Geometry check sheet. Reference: the model listing, model coordinates, mm. Round coordinates to 2 decimals unless told otherwise and drop trailing zeros. Order: outer loops, then holes, each group sorted by start corner. A loop starts at its lowest first (then second) coordinate and runs counter-clockwise, first axis right, second up.
```python
from build123d import *

# Parameters (mm, degrees)
F0_R     = 5
F1_DEPTH = 75
F2_SIZE  = 80


# Not quite as in the source:
# - a feature names something its author has since deleted; it is built from what else it names


with BuildPart() as f1:
    # F0 (on Right) → F1 (new body)
    with BuildSketch(Plane.YZ):
        with BuildLine():
            Line((162.1119900143, -178.1254678004), (19.1804298411, 305.6666666667))
            ThreePointArc((19.1804298411, 305.6666666667), (0, 320), (-19.1804298411, 305.6666666667))
            Line((-19.1804298411, 305.6666666667), (-162.1119900143, -178.1254678004))
            Line((-162.1119900143, -178.1254678004), (162.1119900143, -178.1254678004))
        make_face()
        with Locations((0, -117.917008698)):
            Circle(F0_R, mode=Mode.SUBTRACT)
        Circle(F0_R, mode=Mode.SUBTRACT)
        with Locations((0, 300)):
            Circle(F0_R, mode=Mode.SUBTRACT)
    extrude(amount=F1_DEPTH)

    # F2
    f2_edges = [f1.edges().sort_by_distance(p)[0] for p in [
        (37.5, 162.11199, -178.125468),
        (37.5, -162.11199, -178.125468),
    ]]
    chamfer(f2_edges, length=F2_SIZE)


solid = f1.part
```
(1) Sectioned sample at C-C, the plane x = 5.5. Record the cut outline in (y, z), and give its area (3 significant figures).
Returned:
outline: (-139.45, -101.4) - (-82.11, -178.13) - (82.11, -178.13) - (139.45, -101.4) - (19.18, 305.67) arc R20 ccw to (-19.18, 305.67) - close; hole circle Ø10 at (0, -117.92); hole circle Ø10 at (0, 0); hole circle Ø10 at (0, 300)
area: 81,700 mm2
(2) Sectioned sample at A-A, the plane y = 0. Record the cut outline in (x, z), and give its area (3 significant figures).
Returned:
outline: (0, -178.13) - (75, -178.13) - (75, -122.92) - (0, -122.92) - close; (0, -112.92) - (75, -112.92) - (75, -5) - (0, -5) - close; (0, 5) - (75, 5) - (75, 295) - (0, 295) - close; (0, 305) - (75, 305) - (75, 320) - (0, 320) - close
area: 35,100 mm2
(3) Sectioned sample at D-D, the plane z = 300. Record the cut outline in (x, y).
Returned:
outline: (0, -20.85) - (75, -20.85) - (75, -5) - (0, -5) - close; (0, 5) - (75, 5) - (75, 20.85) - (0, 20.85) - close
(4) Depth check by flat-ended pin: P1, Ø10, axis at x = 46, z = 233.5, coming from the +Y side; P2, Ø12, axis at x = 29, y = -94.5, coming from the -Z side; P3, Ø4, axis at x = 13.5, z = 1.5, coming from the -Y side. Enter the tip coordinate at first touch or a pass-through.
Returned:
P1: stops at y = 41.98
P2: stops at z = -169.58
P3: stops at y = -109.63
(5) Sectioned sample at B-B, the plane z = 0. Record the cut outline in (x, y), and give its area (3 significant figures).
Returned:
outline: (0, -109.49) - (75, -109.49) - (75, -5) - (0, -5) - close; (0, 5) - (75, 5) - (75, 109.49) - (0, 109.49) - close
area: 15,700 mm2
(6) Material ranges on line 1 (Y direction, x = 66.5, z = -122.5); line 2 (Y direction, x = 19, z = 300); line 3 (Y direction, x = 66, z = 93), recorded low to high.
Returned:
line 1: y = -123.68 to -2, 2 to 123.68
line 2: y = -20.85 to -5, 5 to 20.85
line 3: y = -82.01 to 82.01
